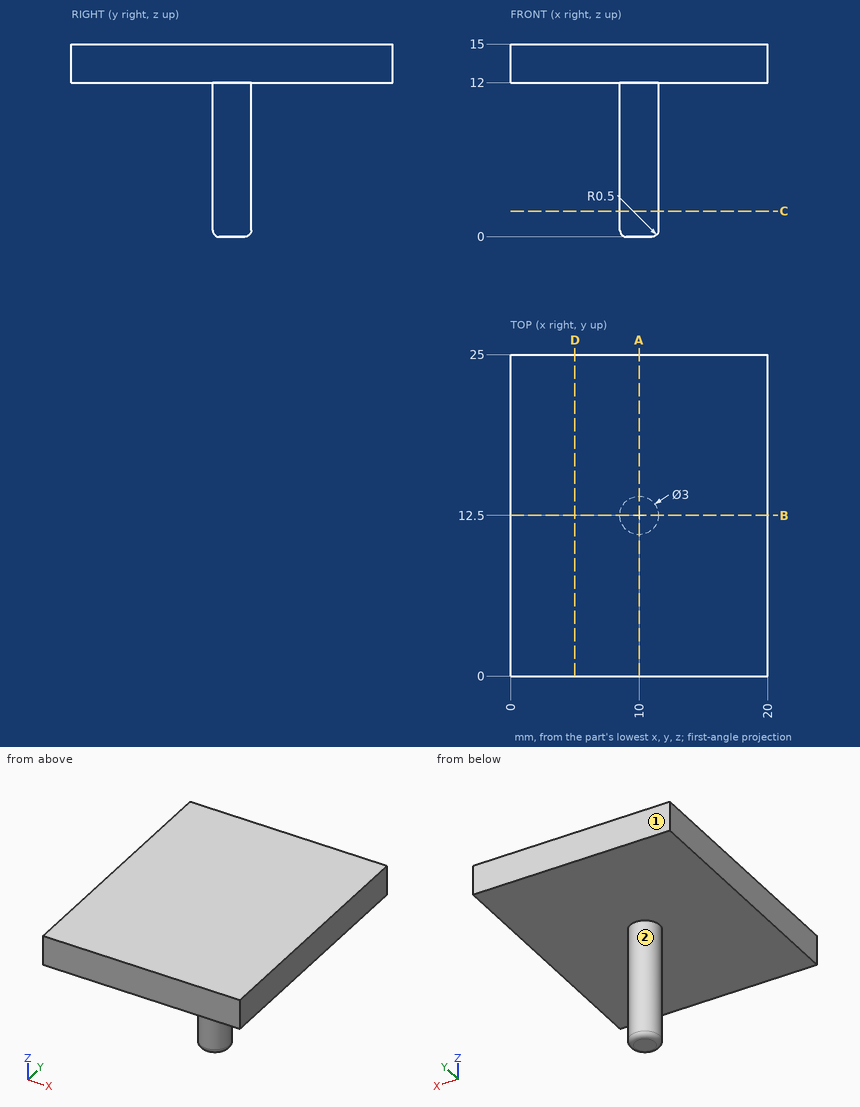
Source: three-view drawing plus pictorial views. Frame: mm from the lowest corner of the part. A direction names the side the tool comes from. Coordinates: 2 decimals unless noted, no trailing zeros. Loops run counter-clockwise (first coordinate to the right, second up) from the corner with the lowest first, then second, coordinate; pieces in that order, holes last. Notation, with made-up numbers: (-35, 18) -> (-10, 18) arc R29 ccw to (-10, 47) -> close; hole circle Ø11 at (38, -33.5). An arc over 180 degrees is marked (long way). Write each question's results on one line, items separated by ' | '. Start each with the question number.
Q1. Section C-C, the plane z = 2. Return the cut outline in (x, y), plus the area to 3 significant figures.
Q2. Ray query, line 1 (Y direction, x = 10, z = 9.5); line 2 (Z direction, x = 7, y = 15.5); line 3 (X direction, y = 11.75, z = 9.25). Return the intervals inside material, ascending. Write a range as from..to.
Q3. Pin query (flat end, axial travel): pin 1 (6 mm diameter, centred on x = 5.5, y = 15, fed in from -Z). Return the tip coordinate at first contact, or that it passes through.
Q4. Section A-A, the plane x = 10. Return the cut outline in (y, z).
Q5. Reachability of the marked faces 1 and 2 from +Z, -Z, +X, -X, +Y, -Y: full face, straight path, thin tool, end or side. Return the list, or none.
Q6. Section B-B, the plane y = 12.5. Return the cut outline in (x, z), plus the area to 3 significant figures.
Q7. Section D-D, the plane x = 5. Return the cut outline in (y, z), plus the area to 3 significant figures.
Found:
1) outline: circle Ø3 at (10, 12.5) | area: 7.07 mm2
2) line 1: 11..14 | line 2: 12..15 | line 3: 8.7..11.3
3) pin 1: z = 12
4) outline: (0, 12) -> (11, 12) -> (11, 0.5) arc R0.5 ccw to (11.5, 0) -> (13.5, 0) arc R0.5 ccw to (14, 0.5) -> (14, 12) -> (25, 12) -> (25, 15) -> (0, 15) -> close
5) face 1: +Z, -Z, +X, -X, +Y | face 2: -Z
6) outline: (0, 12) -> (8.5, 12) -> (8.5, 0.5) arc R0.5 ccw to (9, 0) -> (11, 0) arc R0.5 ccw to (11.5, 0.5) -> (11.5, 12) -> (20, 12) -> (20, 15) -> (0, 15) -> close | area: 95.9 mm2
7) outline: (0, 12) -> (25, 12) -> (25, 15) -> (0, 15) -> close | area: 75.0 mm2
